Geometry: final body of the model. Coordinates: model frame, mm. A direction names the side the tool comes from. Give positions to 0.01 mm unless a question says otherwise; leave off trailing zeros. Order: outer loops, then holes, each group sorted by start corner. A loop starts at its lowest first (then second) coordinate and runs counter-clockwise, first axis right, second up. Notation, with made-up numbers: (84, -34) -> (126, -34) arc R9 ccw to (126, -23) -> close; hole circle Ø6 at (13, 76.5). An arc over 180 degrees is marked (long way). One line per question, with ' | ' between items. Start each with the question number.
(1) Set-up query: faces 4 (the face through (4.88, 34.48, 1.08)), 5 (the face through (-0.94, 19.31, -2.98)), 6 (the face through (0, 36, -2)). Return all of +Z, -Z, +X, -X, +Y, -Y with unobstructed straight access to the full face (end or side cutting, diameter ignored); none if empty.
(2) First-contact query: pin 1 Ø2 at (x, y) = (2, 13) entering from -Z; pin 2 Ø2 at (x, z) = (-0.5, 0.5) entering from +Y; pin 3 Ø1 at (y, z) = (30.5, 0) entering from -X (3 decimals). Flat tips, straight axial feed; report the tip coordinate or a pass-through.
(3) Section A-A (x = 0). Return loops of the section in (y, z) (3 decimals), then the cut area to 3 significant figures.
(4) Section C-C (y = 4). Return loops of the section in (x, z).
(5) Section B-B (y = 13). Return loops of the section in (x, z) (3 decimals), then the cut area to 3 significant figures.
(6) Ray query, L1, parallel to Y at x = -2.75, z = 2.5; L2, parallel to Y at x = -0.25, z = 1; L3, parallel to Z at x = -2, y = 35. Return the intervals inside material, ascending.
(7) Mould query, pull axis Z, two halves, no side actions, for faces 1 (the face through (0, 36, 2)), 2 (the face through (2, 3, 0)), 3 (the face through (3.3, 33, 0.1)). Classes: +Z half, -Z half, draft (parallel to the pull), parting line (faces both ways), or undercut.
```python
from build123d import *

# Parameters (mm, degrees)
CUT_EXTRUDE1_DEPTH = 3
FILLET1_R          = 1


with BuildPart() as part:
    # Sketch1 → Revolve1 (revolve)
    with BuildSketch(Plane.XY, mode=Mode.PRIVATE) as revolve1_sk:
        Polygon((0, 0), (0, 37), (-5, 37), (-5, 33), (-3.125, 33), (-3.125, 6), (-2, 6), (-2, 0), align=None)
    revolve(revolve1_sk.sketch.rotate(Axis((0, 0, 0), (0, 1, 0)), 270), axis=Axis((0, 0, 0), (0, 1, 0)))

    # Sketch3 → Cut-Extrude1 (cut)
    with BuildSketch(Plane(origin=(0, 37, 0), x_dir=(1, 0, 0), z_dir=(0, 1, 0))):
        Polygon((1.154700538, 2), (-1.154700538, 2), (-2.309401077, 0), (-1.154700538, -2), (1.154700538, -2), (2.309401077, 0), align=None)
    extrude(amount=-CUT_EXTRUDE1_DEPTH, mode=Mode.SUBTRACT)

    # Fillet1
    fillet1_edges = [part.edges().sort_by_distance(p)[0] for p in [
        (0, 37, 5),
    ]]
    fillet(fillet1_edges, radius=FILLET1_R)


solid = part.part
```
Response:
1) face 4: +Y, -Y | face 5: -Y | face 6: +Y
2) pin 1: stops at z = -2.96 | pin 2: stops at y = 34 | pin 3: stops at x = -3.125
3) outline: (0, -2) -> (6, -2) -> (6, -3.125) -> (33, -3.125) -> (33, -5) -> (36, -5) arc R1 ccw to (37, -4) -> (37, -2) -> (34, -2) -> (34, 2) -> (37, 2) -> (37, 4) arc R1 ccw to (36, 5) -> (33, 5) -> (33, 3.125) -> (6, 3.125) -> (6, 2) -> (0, 2) -> close | area: 220 mm^2
4) outline: circle Ø4 at (0, 0)
5) outline: circle Ø6.25 at (0, 0) | area: 30.7 mm^2
6) L1: y = 33 to 37 | L2: y = 0 to 34 | L3: z = -4.58 to -0.54, 0.54 to 4.58
7) face 1: undercut | face 2: parting line | face 3: draft
